```python
from build123d import *

# Parameters (mm, degrees)
F0_W        = 6.5
F0_H        = 10
F1_DEPTH    = 7
F3_DEPTH    = 25
F4_W        = 11
F4_H        = 5
F5_DEPTH    = 25
F6_SIZE     = 3
F7_T1_DEPTH = 29.2168298797
F7_T3_DEPTH = 29.2168298797


# Not quite as in the source:
# - a fillet or chamfer that OpenCascade refuses, or shapes differently, is made with other operations: its cross-section is extruded or revolved along the edge and cut away or added
# - a feature names something its author has since deleted; it is built from what else it names


with BuildPart() as f1:
    # F0 (on Top) → F1 (new body)
    with BuildSketch(Plane.XY):
        Polygon((0, 45), (-4, 45), (-4, 30), (0, 22.5), align=None)
        Polygon((4, 45), (0, 45), (0, 22.5), (4, 30), align=None)
        Polygon((-4, 30), (-4, 45), (-5.5, 45), (-12, 45), align=None)
        Polygon((0, -22.5), (-4, -30), (-4, -45), (0, -45), align=None)
        Polygon((4, -30), (0, -22.5), (0, -45), (4, -45), align=None)
        Polygon((12, -45), (4, -30), (4, -45), (5.5, -45), align=None)
        Polygon((-4, -45), (-4, -30), (-12, -45), (-5.5, -45), align=None)
        Polygon((5.5, 45), (4, 45), (4, 30), (12, 45), align=None)
        Polygon((0, 22.5), (-4, 30), (-4, -30), (0, -22.5), (0, 0), align=None)
        Polygon((4, 30), (0, 22.5), (0, 0), (0, -22.5), (4, -30), align=None)
        with Locations((8.75, 50)):
            Rectangle(F0_W, F0_H)
        with Locations((-8.75, 50)):
            Rectangle(F0_W, F0_H)
        with Locations((8.75, -50)):
            Rectangle(F0_W, F0_H)
        with Locations((-8.75, -50)):
            Rectangle(F0_W, F0_H)
    extrude(amount=F1_DEPTH)

    # F2 (on face) → F3 (cut)
    with BuildSketch(Plane(origin=(-12, 0, 0), x_dir=(0, -1, 0), z_dir=(-1, 0, 0))):
        with BuildLine():
            ThreePointArc((-48.4, 3.5), (-50, 5.1), (-51.6, 3.5))
            Line((-51.6, 3.5), (-50, 3.5))
            Line((-50, 3.5), (-48.4, 3.5))
        make_face()
        with BuildLine():
            Line((-50, 3.5), (-51.6, 3.5))
            ThreePointArc((-51.6, 3.5), (-50, 1.9), (-48.4, 3.5))
            Line((-48.4, 3.5), (-50, 3.5))
        make_face()
        with BuildLine():
            ThreePointArc((51.6, 3.5), (50, 5.1), (48.4, 3.5))
            ThreePointArc((48.4, 3.5), (50, 1.9), (51.6, 3.5))
        make_face()
    extrude(amount=-F3_DEPTH, mode=Mode.SUBTRACT)

    # F4 (on face) → F5 (cut)
    with BuildSketch(Plane.XY.offset(7)):
        with Locations((0, -42.5)):
            Rectangle(F4_W, F4_H)
        with Locations((0, 42.5)):
            Rectangle(F4_W, F4_H)
    extrude(amount=-F5_DEPTH, mode=Mode.SUBTRACT)

    # F6
    f6_edges = [f1.edges().sort_by_distance(p)[0] for p in [
        (12, -55, 3.5),
        (-12, -55, 3.5),
        (12, 55, 3.5),
        (-12, 55, 3.5),
    ]]
    chamfer(f6_edges, length=F6_SIZE)

    # F7: chamfer of 5 on 8 edges, made by hand

    # F7_s2 → F7_t1 (cut)
    with BuildSketch(Plane.YZ.offset(-21.8584149398)):
        Polygon((-50, 0), (-55, 5), (-55, 0), align=None)
        Polygon((-50, 7), (-55, 2), (-55, 7), align=None)
        Polygon((50, 7), (55, 2), (55, 7), align=None)
        Polygon((50, 0), (55, 5), (55, 0), align=None)
    extrude(amount=F7_T1_DEPTH, mode=Mode.SUBTRACT)

    # F7_s4 → F7_t3 (cut)
    with BuildSketch(Plane.YZ.offset(-7.3584149398)):
        Polygon((-55, 5), (-50, 0), (-55, 0), align=None)
        Polygon((-55, 2), (-50, 7), (-55, 7), align=None)
        Polygon((50, 7), (55, 2), (55, 7), align=None)
        Polygon((50, 0), (55, 5), (55, 0), align=None)
    extrude(amount=F7_T3_DEPTH, mode=Mode.SUBTRACT)


solid = f1.part
```
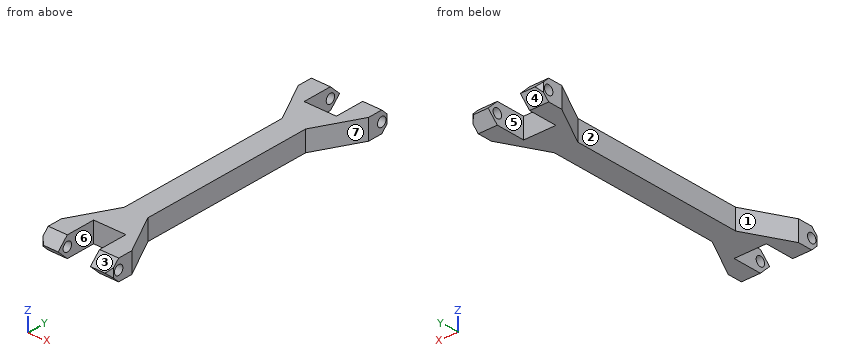
Read the model definition and answer for the solid it produces. Units are mm, in the model's axes. Face numbers are marked on the shaded views. A direction names the side the tool comes from. Give positions to 0.01 mm unless a question says otherwise; leave off trailing zeros. Write each loop counter-clockwise with the first axis right and the second up, starting at its lowest first coordinate (ties: lowest second). Pieces come first, ordered by that corner, then holes. Notation, with made-up numbers: (5.25, 2.5) - (29.25, 2.5) arc R37 ccw to (29.25, 39.5) - close; hole circle Ø11 at (67.25, 61). An arc over 180 degrees is marked (long way). Write item = value, one per line. Start each with the question number.
Item 1: Find section B-B (y = 41.5). Give the vertices of the cut face in (x, z).
Item 2: A tool of negligible diameter and unlimited length cuts with its end or side. For the marked faces 5, 6 and 7, from which of +Z, -Z, +X, -X, +Y, -Y can it reach the whole face along a straight path? Write none if from no direction.
Item 3: Find section C-C (y = 2). Give the vertices of the cut face in (x, z), then the cut area to 3 significant figures.
Item 4: Find section A-A (x = -7.75). Give the vertices of the cut face in (y, z).
Item 5: Each of these flat-tipped pins is pushed along its axis until it touches: P1, Ø1.5, axis at x = 4, z = 2, coming from the +Y side; P2, Ø1.5, axis at x = -9, z = 5, coming from the +Y side; P3, Ø2.5, axis at y = -50, z = 3.5, coming from the -X side; P4, Ø3.5, axis at y = -6, z = 4, coming from the +X side. Where does it stop, or does it pass through?
Item 6: Find the intervals of material crossed by probe 1 along Z at (x, y) = (9, 50); probe 2 along X at (y, z) = (-46.5, 5.75); probe 3 along X at (y, z) = (4, 2), in increasing order. Write a range as [from, to].
Item 7: The mould has two halves that part along Y. Classify the marked faces 1, 2, 3 and 4: +Y half, -Y half, draft (parallel to the pull), parting line (faces both ways), or undercut.
Response:
q1.outline = (-10.13, 0) - (-5.5, 0) - (-5.5, 7) - (-10.13, 7) - close; (5.5, 0) - (10.13, 0) - (10.13, 7) - (5.5, 7) - close
q2.face_5 = +Z, -Z, +Y
q2.face_6 = +Z, -Z, -Y
q2.face_7 = +Z, -Z, +X
q3.outline = (-4, 0) - (4, 0) - (4, 7) - (-4, 7) - close
q3.area = 56.0 mm²
q4.outline = (-53.5, 3.5) - (-50, 0) - (-37.03, 0) - (-37.03, 7) - (-50, 7) - close; (37.03, 0) - (50, 0) - (53.5, 3.5) - (50, 7) - (37.03, 7) - close; hole circle Ø3.2 at (-50, 3.5); hole circle Ø3.2 at (50, 3.5)
q5.P1 = 40
q5.P2 = 52.75
q5.P3 = through
q5.P4 = 4
q6.probe_1 = [0, 1.9], [5.1, 7]
q6.probe_2 = [-12, -5.5], [5.5, 12]
q6.probe_3 = [-4, 4]
q7.face_1 = undercut
q7.face_2 = undercut
q7.face_3 = -Y half
q7.face_4 = +Y half
